Check sheet for the modelled part. Datum: model origin and axes. Units: mm. Round coordinates to 2 decimals unless told otherwise and drop trailing zeros. Write each loop counter-clockwise with the first axis right and the second up, starting at its lowest first coordinate (ties: lowest second). Pieces come first, ordered by that corner, then holes. Notation, with made-up numbers: (79.25, 57.5) - (89.25, 57.5) arc R25 ccw to (89.25, 94.5) - close; hole circle Ø9 at (60.25, 41). An arc over 180 degrees is marked (long way). Answer as a JSON object with one key per item and string values. Group by question number.
Item 1: Sectioned sample at B-B on y = 1. Record the boundary of the cut face in (x, z), plus the area to 3 significant figures.
Item 2: Sectioned sample at C-C on z = 52. Record the boundary of the cut face in (x, y).
Item 3: Sectioned sample at A-A on z = 85. Record the boundary of the cut face in (x, y), plus the area to 3 significant figures.
Item 4: Gauge pin test, flat ends, axial feed: P1, Ø1.5, axis at y = 2, z = 1.5, coming from the +X side; P2, Ø0.9, axis at x = 1, y = 1.5, coming from the -Z side. Record the tip position at first contact, or that the pin passes through.
Item 5: Thickness scan on line 1 (Z direction, x = 3, y = 2.2); line 2 (Z direction, x = -4.25, y = 1.85); line 3 (X direction, y = 2.65, z = -56.5). Record the ranges inside material, lowest first.
Autodesk Inventor part; units mm, degrees
ref_plane "YZ Plane" through (0, 0, 0) normal (1, 0, 0) x (0, 1, 0)
ref_plane "XZ Plane" through (0, 0, 0) normal (0, 1, 0) x (-1, 0, 0)
ref_plane "XY Plane" through (0, 0, 0) normal (0, 0, 1) x (1, 0, 0)
sketch "草圖1" plane through (0, 0, 0) normal (0, 1, 0) x (-1, 0, 0)
  line L0 (0, 80) -> (9, 80)
  line L1 (9, 80) -> (9, -80)
  line L2 (9, -80) -> (0, -80)
  line L3 (0, -80) -> (0, 80)
  line L4 (7, 4.5) -> (2, 4.5)
  line L5 (2, 4.5) -> (2, -4.5)
  line L6 (2, -4.5) -> (7, -4.5)
  line L7 (7, -4.5) -> (7, 4.5)
  line L8 (9, 80) -> (9, 90)
  line L9 (9, 90) -> (-3, 90)
  line L10 (-8, 85) -> (-8, 85)
  line L11 (-3, 80) -> (0, 80)
  arc A0 (-8, 85) -> (-3, 80) centre (-3, 85) ccw
  arc A1 (-3, 90) -> (-8, 85) centre (-3, 85) ccw
  circle A2 centre (-3, 85) radius 2.5
  line L12 (9, 0) -> (0, 0)
  line L13 (9, -80) -> (9, -90)
  line L14 (9, -90) -> (-3, -90)
  line L15 (-3, -80) -> (0, -80)
  arc A3 (-3, -80) -> (-8, -85) centre (-3, -85) ccw
  arc A4 (-8, -85) -> (-3, -90) centre (-3, -85) ccw
  circle A5 centre (-3, -85) radius 2.5
  line L16 (9, 90) -> (0, 90)
  line L17 (0, 90) -> (0, 100)
  line L18 (0, 100) -> (9, 100)
  line L19 (9, 100) -> (9, 90)
  line L20 (9, -90) -> (0, -90)
  line L21 (0, -90) -> (0, -100)
  line L22 (0, -100) -> (9, -100)
  line L23 (9, -100) -> (9, -90)
  line L24 (7, 97) -> (2, 97)
  line L25 (2, 97) -> (2, 88)
  line L26 (2, 88) -> (7, 88)
  line L27 (7, 88) -> (7, 97)
  line L28 (7, -97) -> (2, -97)
  line L29 (2, -97) -> (2, -88)
  line L30 (2, -88) -> (7, -88)
  line L31 (7, -88) -> (7, -97)
  point P0 (7, 0)
  point P1 (4.5, 4.5)
  point P2 (4.5, 80)
  point P3 (-8, 90)
  point P4 (-8, -90)
  point P5 (-8, -85)
  point P6 (0, -90)
  point P7 (4.5, 97)
  point P8 (4.5, 100)
  point P9 (4.5, -97)
  dimension "d0" = 160
  dimension "d1" = 9
  dimension "d2" = 9
  dimension "d3" = 5
  dimension "d4" = 10
  dimension "d5" = 17
  dimension "d6" = 5
  dimension "d7" = 5
  dimension "d8" = 5
  dimension "d11" = 10
  dimension "d12" = 9
  dimension "d13" = 9
  dimension "d14" = 10
  dimension "d15" = 5
  dimension "d16" = 9
  dimension "d17" = 3
extrude "擠出1" add sketch "草圖1" along normal blind 3 contours L11 A0 A1 L9 L25 L26 L27 L8 L0 | L0 L1 L12 L7 L4 L5 L3 | L12 L5 L6 L7 L1 L2 L3 | L9 L27 L24 L25 L17 L18 L19 | L2 L13 L14 L31 L30 L29 A4 A3 L15 | L23 L22 L21 L14 L29 L28 L31
properties part number "upper_Bar" material "MDF Medium Density Fiberboard"
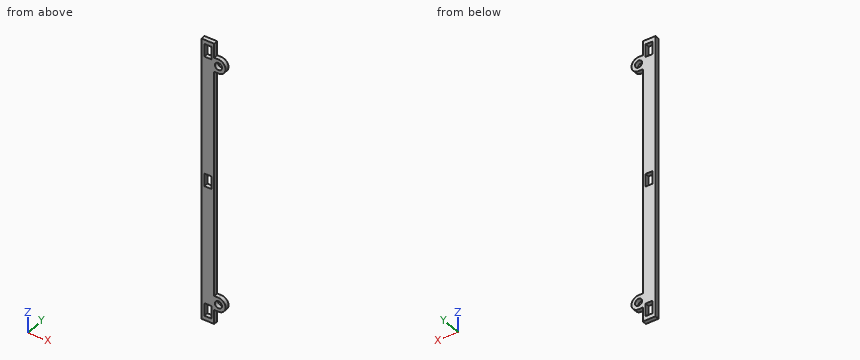
Completed:
{
 "1": {"outline": "(-9, -100) - (0, -100) - (0, -90) - (3, -90) arc R5 ccw to (3, -80) - (0, -80) - (0, 80) - (3, 80) arc R5 ccw to (3, 90) - (0, 90) - (0, 100) - (-9, 100) - close; hole (-7, -97) - (-2, -97) - (-2, -88) - (-7, -88) - close; hole (-7, -4.5) - (-2, -4.5) - (-2, 4.5) - (-7, 4.5) - close; hole (-7, 88) - (-2, 88) - (-2, 97) - (-7, 97) - close; hole circle Ø5 at (3, -85); hole circle Ø5 at (3, 85)", "area": "1,760 mm²"},
 "2": {"outline": "(-9, 0) - (0, 0) - (0, 3) - (-9, 3) - close"},
 "3": {"outline": "(-9, 0) - (0.5, 0) - (0.5, 3) - (-9, 3) - close; (5.5, 0) - (8, 0) - (8, 3) - (5.5, 3) - close", "area": "36.0 mm²"},
 "4": {"P1": "x = 0", "P2": "z = -90"},
 "5": {"line 1": "-90 to -87.5, -82.5 to -80, 80 to 82.5, 87.5 to 90", "line 2": "-100 to -97, -88 to -4.5, 4.5 to 88, 97 to 100", "line 3": "-9 to 0"}
}
